Geometry: final body of the model. Coordinates: model frame, mm. Face numbers are marked on the shaded views. A direction names the side the tool comes from. Round coordinates to 2 decimals unless told otherwise and drop trailing zeros. Loops run counter-clockwise (first coordinate to the right, second up) from the corner with the lowest first, then second, coordinate; pieces in that order, holes last. Notation, with made-up numbers: (72.25, 46) -> (99.25, 46) arc R20 cw to (99.25, 77) -> close; hole circle Ø8 at (9, -27). An arc over 180 degrees is marked (long way). Answer in a Markdown table with one row per item.
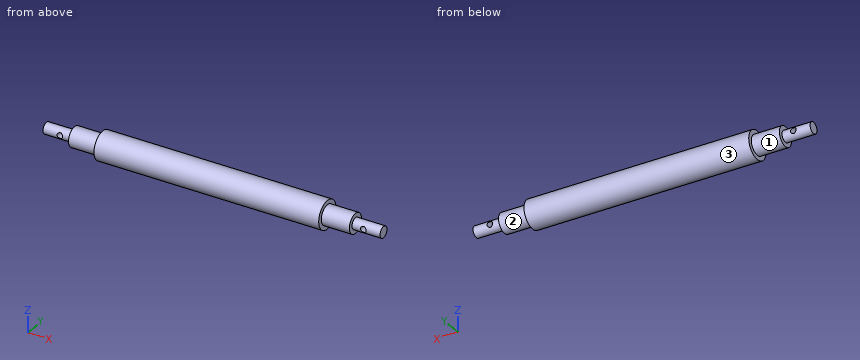
```python
from build123d import *

# Parameters (mm, degrees)
F0_R      = 25
F1_DEPTH  = 200
F2_R      = 10
F3_DEPTH  = 100
F4_R      = 10
F5_DEPTH  = 100
F6_R      = 5
F7_DEPTH  = 50
F8_R      = 17.5
F9_DEPTH  = 50
F10_R     = 17.5
F11_DEPTH = 50


with BuildPart() as f1:
    # F0 (on Right) → F1 (new body, symmetric)
    with BuildSketch(Plane.YZ):
        Circle(F0_R)
    extrude(amount=F1_DEPTH, both=True)

    # F2 (on face) → F3 (join)
    with BuildSketch(Plane(origin=(-200, 0, 0), x_dir=(0, -1, 0), z_dir=(-1, 0, 0))):
        Circle(F2_R)
    extrude(amount=F3_DEPTH)

    # F4 (on face) → F5 (join)
    with BuildSketch(Plane.YZ.offset(200)):
        Circle(F4_R)
    extrude(amount=F5_DEPTH)

    # F6 (on Front) → F7 (cut, symmetric)
    with BuildSketch(Plane.XZ):
        with Locations((270, 0)):
            Circle(F6_R)
        with Locations((-270, 0)):
            Circle(F6_R)
    extrude(amount=F7_DEPTH, both=True, mode=Mode.SUBTRACT)

    # F8 (on face) → F9 (join)
    with BuildSketch(Plane(origin=(-200, 0, 0), x_dir=(0, -1, 0), z_dir=(-1, 0, 0))):
        Circle(F8_R)
    extrude(amount=F9_DEPTH)

    # F10 (on face) → F11 (join)
    with BuildSketch(Plane.YZ.offset(200)):
        Circle(F10_R)
    extrude(amount=F11_DEPTH)


solid = f1.part
```
Item 1: Section query B-B, the plane y = 0. Output: boundary loops of the cut face in (x, z), and give its area (3 significant figures).
Ans:
| item | result |
|---|---|
| outline | (-300, -10) -> (-250, -10) -> (-250, -17.5) -> (-200, -17.5) -> (-200, -25) -> (200, -25) -> (200, -17.5) -> (250, -17.5) -> (250, -10) -> (300, -10) -> (300, 10) -> (250, 10) -> (250, 17.5) -> (200, 17.5) -> (200, 25) -> (-200, 25) -> (-200, 17.5) -> (-250, 17.5) -> (-250, 10) -> (-300, 10) -> close; hole circle Ø10 at (-270, 0); hole circle Ø10 at (270, 0) |
| area | 25,300 mm2 |
Item 2: Section query A-A, the plane z = 0. Output: boundary loops of the cut face in (x, y), and give its area (3 significant figures).
Ans:
| item | result |
|---|---|
| outline | (-300, -10) -> (-275, -10) -> (-275, 10) -> (-300, 10) -> close; (-265, -10) -> (-250, -10) -> (-250, -17.5) -> (-200, -17.5) -> (-200, -25) -> (200, -25) -> (200, -17.5) -> (250, -17.5) -> (250, -10) -> (265, -10) -> (265, 10) -> (250, 10) -> (250, 17.5) -> (200, 17.5) -> (200, 25) -> (-200, 25) -> (-200, 17.5) -> (-250, 17.5) -> (-250, 10) -> (-265, 10) -> close; (275, -10) -> (300, -10) -> (300, 10) -> (275, 10) -> close |
| area | 25,100 mm2 |
Item 3: Ray query, L1, parallel to X at y = -0.75, z = 0; L2, parallel to Z at x = 270, y = 0.25; L3, parallel to X at y = -11, z = 14. Return the intervals inside material, ascending.
Ans:
| item | result |
|---|---|
| L1 | -300 to -275, -265 to 265, 275 to 300 |
| L2 | -10 to -5, 5 to 10 |
| L3 | -200 to 200 |
Item 4: Section query D-D, the plane x = -270. Output: boundary loops of the cut face in (y, z).
Ans:
| item | result |
|---|---|
| outline | (-8.66, -5) arc R10 ccw to (8.66, -5) -> close; (-8.66, 5) -> (8.66, 5) arc R10 ccw to start |
Item 5: Set-up query: the marked faces 1, 2 and 3. Return all of +Z, -Z, +X, -X, +Y, -Y with unobstructed straight access to the full face (end or side cutting, diameter ignored); none if empty.
Ans:
| item | result |
|---|---|
| face 1 | -X |
| face 2 | +X |
| face 3 | +X, -X |
Item 6: Section query C-C, the plane x = 27. Output: boundary loops of the cut face in (y, z).
Ans:
| item | result |
|---|---|
| outline | circle Ø50 at (0, 0) |
Item 7: First-contact query: P1, Ø10.5, axis at y = -7, z = 8, coming from the -X side; P2, Ø8, axis at y = -19.5, z = 12.5, coming from the +X side; P3, Ø3, axis at x = 32, z = 3, coming from the -Y side; P4, Ø5, axis at y = -16, z = -2, coming from the +X side. Flat tips, straight axial feed; report the tip coordinate or a pass-through.
Ans:
| item | result |
|---|---|
| P1 | x = -300 |
| P2 | x = 200 |
| P3 | y = -24.95 |
| P4 | x = 250 |
